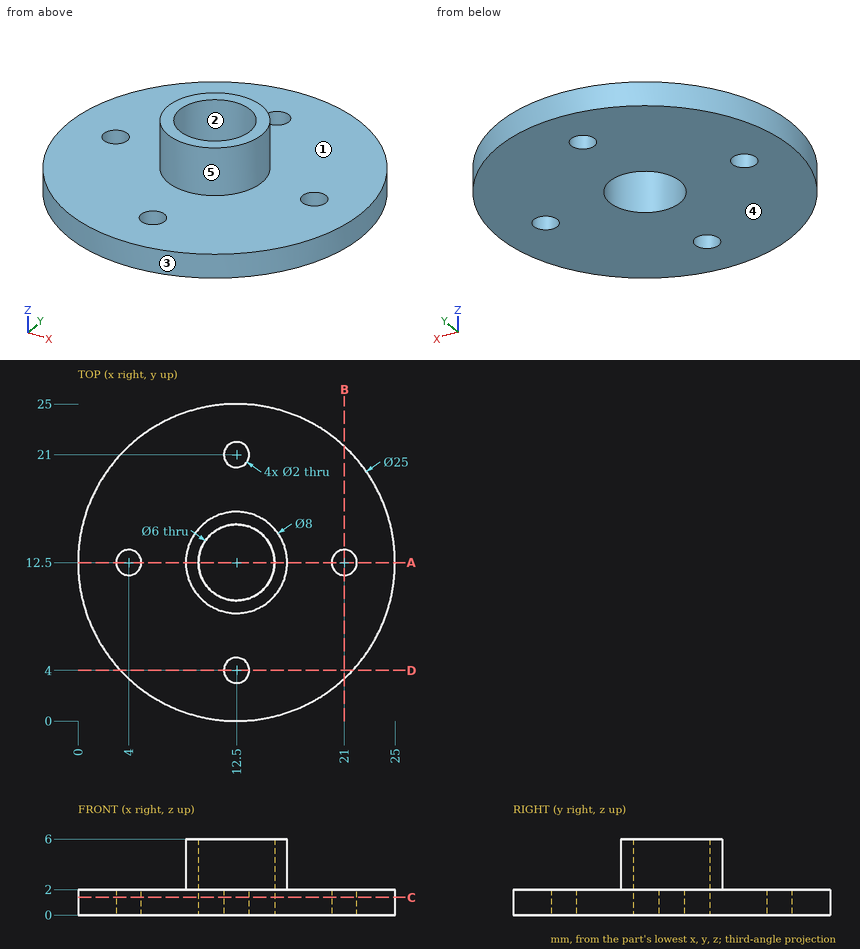
Design review of the part shown in the three views and the two pictorial views. Dimensions are in mm from the part's minimum x, y and z. A direction names the side the tool comes from. Give positions to 0.01 mm unless a question says otherwise; leave off trailing zeros. Loops run counter-clockwise (first coordinate to the right, second up) from the corner with the lowest first, then second, coordinate; pieces in that order, holes last. Notation, with made-up numbers: M 0.25,-16.5 L 36.25,-16.5 A23 cw 36.25,5.5 Z; hole C 14,22.25 d10. An arc over 180 degrees is marked long. Answer as a JSON object with one key per item and string values. Group by question number.
Q1. Add section B-B on x = 21. Give the boundary of the cut face in (y, z), and give its area (3 significant figures).
Q2. Add section C-C on z = 1.4. Give the boundary of the cut face in (x, y).
Q3. Mouldability with a two-part tool opening along Y and no side actions: class the marked faces 1, 2 and 3 as +Y half, -Y half, draft (parallel to the pull), parting line (faces both ways), or undercut.
Q4. Add section A-A on y = 12.5. Give the boundary of the cut face in (x, z), and give its area (3 significant figures).
Q5. Tool access review of the marked faces 4 and 5: name each direction out of +Z, -Z, +X, -X, +Y, -Y from which nothing blocks a thin tool from reaching the whole face with its end or side.
Q6. Insertion check: P1, Ø12.5, axis at x = 15.5, y = 16, coming from the +Z side; P2, Ø2, axis at x = 8.5, y = 8, coming from the +Z side. Each pin has a flat end and moves straight along its axis. Give the tip position at first contact, or say it passes through.
Q7. For probe 1 along Y at (x, z) = (12.5, 0.55); probe 2 along Z at (x, y) = (15.25, 8); probe 3 along X at (y, z) = (12.75, 1.5), list the stretches that pass through material, from the lowest coordinate up. Write a range as [from, to].
Checked values:
{
 "1": {"outline": "M 3.33,0 L 11.5,0 L 11.5,2 L 3.33,2 Z; M 13.5,0 L 21.67,0 L 21.67,2 L 13.5,2 Z", "area": "32.7 mm²"},
 "2": {"outline": "C 12.5,12.5 d25; hole C 4,12.5 d2; hole C 12.5,12.5 d6; hole C 12.5,4 d2; hole C 12.5,21 d2; hole C 21,12.5 d2"},
 "3": {"face 1": "draft", "face 2": "undercut", "face 3": "parting line"},
 "4": {"outline": "M 0,0 L 3,0 L 3,2 L 0,2 Z; M 5,0 L 9.5,0 L 9.5,6 L 8.5,6 L 8.5,2 L 5,2 Z; M 15.5,0 L 20,0 L 20,2 L 16.5,2 L 16.5,6 L 15.5,6 Z; M 22,0 L 25,0 L 25,2 L 22,2 Z", "area": "38.0 mm²"},
 "5": {"face 4": "-Z, +X, -X, +Y, -Y", "face 5": "+Z"},
 "6": {"P1": "z = 6", "P2": "z = 2"},
 "7": {"probe 1": "[0, 3], [5, 9.5], [15.5, 20], [22, 25]", "probe 2": "[0, 2]", "probe 3": "[0, 3.03], [4.97, 9.51], [15.49, 20.03], [21.97, 25]"}
}
